Input: part model. Units: mm. Frame: model coordinates. A direction names the side the tool comes from. Coordinates: 2 decimals unless noted, no trailing zeros. Order: outer loops, then holes, each group sorted by start corner. A loop starts at its lowest first (then second) coordinate and runs counter-clockwise, first axis right, second up. Notation, with made-up numbers: (-14, 86) -> (41, 86) arc R22 ccw to (41, 121) -> close; hole circle Ø6 at (-28.75, 31). An arc over 180 degrees is marked (long way). One line per question, with ' | ' between items.
```python
from build123d import *
from OCP.BRepFilletAPI import BRepFilletAPI_MakeChamfer

# Parameters (mm, degrees)
BOSS_EXTRUDE1_DEPTH                                 = 3.5
CSK_FOR_M3_COUNTERSUNK_FLAT_HEAD_SCREW1_D           = 3.6
CSK_FOR_M3_COUNTERSUNK_FLAT_HEAD_SCREW1_CSINK_D     = 7
CSK_FOR_M3_COUNTERSUNK_FLAT_HEAD_SCREW1_CSINK_ANGLE = 90
CHAMFER1_SIZE                                       = 2.5
CHAMFER1_SIZE2                                      = 1.443375673
FILLET2_R                                           = 2
SKETCH4_W                                           = 14
SKETCH4_H                                           = 4.115813757
CUT_EXTRUDE1_DEPTH                                  = 43.570529862
CUT_EXTRUDE1_DEPTH_BACK                             = 15
BODY_MOVE_COPY1_ANGLE                               = 180


with BuildPart() as part:
    # Sketch1 → Boss-Extrude1 (new body)
    with BuildSketch(Plane.XY):
        with BuildLine():
            Line((-20, 30), (20, 30))
            ThreePointArc((20, 30), (27.071067812, 27.071067812), (30, 20))
            Line((30, 20), (30, -20))
            ThreePointArc((30, -20), (27.071067812, -27.071067812), (20, -30))
            Line((20, -30), (-20, -30))
            ThreePointArc((-20, -30), (-27.071067812, -27.071067812), (-30, -20))
            Line((-30, -20), (-30, 20))
            ThreePointArc((-30, 20), (-27.071067812, 27.071067812), (-20, 30))
        make_face()
    extrude(amount=BOSS_EXTRUDE1_DEPTH)

    # CSK for M3 Countersunk Flat Head Screw1 (through all)
    with Locations(Plane.XY.offset(3.5)):
        with Locations((-20, 20), (20, 20), (20, -20), (-20, -20)):
            CounterSinkHole(CSK_FOR_M3_COUNTERSUNK_FLAT_HEAD_SCREW1_D / 2, CSK_FOR_M3_COUNTERSUNK_FLAT_HEAD_SCREW1_CSINK_D / 2, counter_sink_angle=CSK_FOR_M3_COUNTERSUNK_FLAT_HEAD_SCREW1_CSINK_ANGLE)

    # Chamfer1: one chamfer whose edges measure the first distance from different faces: ONE call of the kernel's chamfer builder (chamfer() names one face for all edges)
    chamfer1_edges_1 = [part.edges().sort_by_distance(p)[0] for p in [
        (-27.071067812, 27.071067812, 3.5),
    ]]
    chamfer1_side_1 = [part.faces().sort_by_distance(p)[0] for p in [
        (-27.071067812, 27.071067812, 1.75),
    ]]
    chamfer1_edges_2 = [part.edges().sort_by_distance(p)[0] for p in [
        (-30, 0, 3.5),
    ]]
    chamfer1_side_2 = [part.faces().sort_by_distance(p)[0] for p in [
        (-30, 0, 1.75),
    ]]
    chamfer1_edges_3 = [part.edges().sort_by_distance(p)[0] for p in [
        (-27.071067812, -27.071067812, 3.5),
    ]]
    chamfer1_side_3 = [part.faces().sort_by_distance(p)[0] for p in [
        (-27.071067812, -27.071067812, 1.75),
    ]]
    chamfer1_edges_4 = [part.edges().sort_by_distance(p)[0] for p in [
        (0, -30, 3.5),
    ]]
    chamfer1_side_4 = [part.faces().sort_by_distance(p)[0] for p in [
        (0, -30, 1.75),
    ]]
    chamfer1_edges_5 = [part.edges().sort_by_distance(p)[0] for p in [
        (27.071067812, -27.071067812, 3.5),
    ]]
    chamfer1_side_5 = [part.faces().sort_by_distance(p)[0] for p in [
        (27.071067812, -27.071067812, 1.75),
    ]]
    chamfer1_edges_6 = [part.edges().sort_by_distance(p)[0] for p in [
        (30, 0, 3.5),
    ]]
    chamfer1_side_6 = [part.faces().sort_by_distance(p)[0] for p in [
        (30, 0, 1.75),
    ]]
    chamfer1_edges_7 = [part.edges().sort_by_distance(p)[0] for p in [
        (27.071067812, 27.071067812, 3.5),
    ]]
    chamfer1_side_7 = [part.faces().sort_by_distance(p)[0] for p in [
        (27.071067812, 27.071067812, 1.75),
    ]]
    chamfer1_edges_8 = [part.edges().sort_by_distance(p)[0] for p in [
        (0, 30, 3.5),
    ]]
    chamfer1_side_8 = [part.faces().sort_by_distance(p)[0] for p in [
        (0, 30, 1.75),
    ]]
    chamfer1 = BRepFilletAPI_MakeChamfer(part.part.solid().wrapped)
    for e in chamfer1_edges_1:
        chamfer1.Add(CHAMFER1_SIZE, CHAMFER1_SIZE2, e.wrapped, chamfer1_side_1[0].wrapped)  # the first distance lies on this face
    for e in chamfer1_edges_2:
        chamfer1.Add(CHAMFER1_SIZE, CHAMFER1_SIZE2, e.wrapped, chamfer1_side_2[0].wrapped)  # the first distance lies on this face
    for e in chamfer1_edges_3:
        chamfer1.Add(CHAMFER1_SIZE, CHAMFER1_SIZE2, e.wrapped, chamfer1_side_3[0].wrapped)  # the first distance lies on this face
    for e in chamfer1_edges_4:
        chamfer1.Add(CHAMFER1_SIZE, CHAMFER1_SIZE2, e.wrapped, chamfer1_side_4[0].wrapped)  # the first distance lies on this face
    for e in chamfer1_edges_5:
        chamfer1.Add(CHAMFER1_SIZE, CHAMFER1_SIZE2, e.wrapped, chamfer1_side_5[0].wrapped)  # the first distance lies on this face
    for e in chamfer1_edges_6:
        chamfer1.Add(CHAMFER1_SIZE, CHAMFER1_SIZE2, e.wrapped, chamfer1_side_6[0].wrapped)  # the first distance lies on this face
    for e in chamfer1_edges_7:
        chamfer1.Add(CHAMFER1_SIZE, CHAMFER1_SIZE2, e.wrapped, chamfer1_side_7[0].wrapped)  # the first distance lies on this face
    for e in chamfer1_edges_8:
        chamfer1.Add(CHAMFER1_SIZE, CHAMFER1_SIZE2, e.wrapped, chamfer1_side_8[0].wrapped)  # the first distance lies on this face
    add(Compound.cast(chamfer1.Shape()), mode=Mode.REPLACE)

    # Fillet2
    fillet2_edges = [part.edges().sort_by_distance(p)[0] for p in [
        (0, -30, 1),
        (27.071067812, -27.071067812, 1),
        (-27.071067812, -27.071067812, 1),
        (30, 0, 1),
        (-30, 0, 1),
        (27.071067812, 27.071067812, 1),
        (-27.071067812, 27.071067812, 1),
        (0, 30, 1),
    ]]
    fillet(fillet2_edges, radius=FILLET2_R)

    # Sketch4 → Cut-Extrude1 (cut, two sides)
    with BuildSketch(Plane(origin=(0, 0, 0), x_dir=(1, 0, 0), z_dir=(0, 1, 0))) as cut_extrude1_sk:
        with Locations((0, 1.057906879)):
            Rectangle(SKETCH4_W, SKETCH4_H)
    extrude(amount=CUT_EXTRUDE1_DEPTH, mode=Mode.SUBTRACT)
    extrude(cut_extrude1_sk.sketch, amount=-CUT_EXTRUDE1_DEPTH_BACK, mode=Mode.SUBTRACT)


with BuildPart() as part_1:
    # Body-Move/Copy1: moved
    add(part.part.rotate(Axis((0, 0, 1.75), (0, 1, 0)), BODY_MOVE_COPY1_ANGLE))


solid = part_1.part
```
1. Mould query, pull axis X, two halves, no side actions, for faces 3 (the face through (-26.21, 26.34, 0.55)), 4 (the face through (27.15, 26.99, 3.27)), 5 (the face through (0, 0, 0)), 6 (the face through (20.968, 21.518, 2.613)). Classes: released by +X, released by -X, zero draft, split by the parting line, or undercut.
Recorded:
face 3: released by -X | face 4: released by +X | face 5: zero draft | face 6: undercut
2. Cut plane C-C, the plane x = 4.5. Return loops of the section in (y, z), and give its area (3 significant figures).
Recorded:
outline: (-30, 3.04) arc R2 ccw to (-29.73, 2.04) -> (-28.56, 0) -> (28.56, 0) -> (29.73, 2.04) arc R2 ccw to (29.93, 2.5) -> (-15, 2.5) -> (-15, 3.5) -> (-30, 3.5) -> close | area: 161 mm^2
3. Ray query, line 1 (X direction, y = 7, z = 3.1); line 2 (X direction, y = -20, z = 2.75); line 3 (Y direction, x = -20, z = 2.15). Return the intervals inside material, ascending. Write a range as [from, to].
Recorded:
line 1: x = [-30, -7], [7, 30] | line 2: x = [-29.98, -21.8], [-18.2, 18.2], [21.8, 29.98] | line 3: y = [-29.79, -21.8], [-18.2, 18.2], [21.8, 29.79]
4. Pin query (flat end, axial travel): pin 1 Ø1.5 at (x, y) = (-18.5, 20) entering from +Z; pin 2 Ø6 at (x, y) = (20, 20) entering from -Z; pin 3 Ø2 at (x, y) = (-20, -20) entering from +Z; pin 4 Ø4 at (x, y) = (1.5, 14.5) entering from +Z. Return the tip coordinate at first contact, or that it passes through.
Recorded:
pin 1: stops at z = 3.5 | pin 2: stops at z = 0.5 | pin 3: passes through | pin 4: stops at z = 2.5
5. Cut plane B-B, the plane x = -11. Return loops of the section in (y, z).
Recorded:
outline: (-30, 3.04) arc R2 ccw to (-29.73, 2.04) -> (-28.56, 0) -> (28.56, 0) -> (29.73, 2.04) arc R2 ccw to (30, 3.04) -> (30, 3.5) -> (-30, 3.5) -> close
6. Access query for faces 1 (the face through (19.766, -18.215, 2.613)), 2 (the face through (0, 7, 2.5)). Directions: +Z, -Z, +X, -X, +Y, -Y. A direction counts if a zero-diameter tool reaches every point of the face in a straight line with its end or side. Return the directions, or none.
Recorded:
face 1: +Z, -Z | face 2: +Z, +Y
7. Cut plane A-A, the plane y = 0.5. Return loops of the section in (x, z).
Recorded:
outline: (-30, 3.04) arc R2 ccw to (-29.73, 2.04) -> (-28.56, 0) -> (28.56, 0) -> (29.73, 2.04) arc R2 ccw to (30, 3.04) -> (30, 3.5) -> (7, 3.5) -> (7, 2.5) -> (-7, 2.5) -> (-7, 3.5) -> (-30, 3.5) -> close
